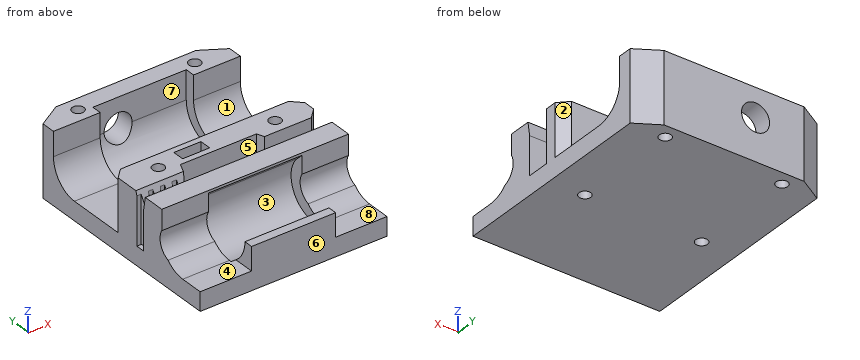
from build123d import *

# Parameters (mm, degrees)
SKETCH1_W                = 40
SKETCH1_H                = 48
BOSS_EXTRUDE1_DEPTH      = 4
BOSS_EXTRUDE2_DEPTH      = 11.15
BOSS_EXTRUDE2_DEPTH_BACK = 4
SKETCH5_W                = 40
SKETCH5_H                = 5.225
SKETCH5_W_2              = 18
SKETCH5_H_2              = 5
SKETCH5_H_3              = 6
FILLET1_DEPTH            = 40
SKETCH6_R                = 1.25
CUT_EXTRUDE4_DEPTH       = 58.214705278
CHAMFER2_SIZE            = 2
CHAMFER3_SIZE            = 3
CHAMFER3_SIZE2           = 1
CHAMFER4_SIZE            = 3
CHAMFER4_SIZE2           = 0.5
CUT_EXTRUDE6_DEPTH       = 10
CUT_EXTRUDE6_DEPTH_BACK  = 10
CUT_EXTRUDE8_REACH       = 66.292
SKETCH12_R               = 3
SKETCH13_R               = 1.5
CUT_EXTRUDE10_DEPTH      = 10.275
CUT_EXTRUDE7_DEPTH       = 1.25
CUT_EXTRUDE7_DEPTH_BACK  = 1.25
CHAMFER5_SIZE            = 5
CHAMFER5_SIZE2           = 3
CHAMFER6_SIZE            = 3
CHAMFER6_SIZE2           = 5
CUT_EXTRUDE12_DEPTH      = 46.535947422
CUT_EXTRUDE12_DEPTH_BACK = 46.535947422
SKETCH15_R               = 3.5


with BuildPart() as part:
    # Sketch1 → Boss-Extrude1 (new body)
    with BuildSketch(Plane.XY):
        with Locations((20, 14)):
            Rectangle(SKETCH1_W, SKETCH1_H)
    extrude(amount=BOSS_EXTRUDE1_DEPTH)

    # Sketch5 → Boss-Extrude2 (add, two sides: drawn at the far end of the back side and taken through both)
    with BuildSketch(Plane.XY.offset(4).offset(-BOSS_EXTRUDE2_DEPTH_BACK)):
        Polygon((0.9, 8.125), (0, 8.125), (0, 15.5), (40, 15.5), (40, 9), (28, 9), (27.357142857, 10.5), (11.081237185, 10.5), (9.763380042, 7.425), (8.800403155, 7.425), (8.500403155, 8.125), (7.531690021, 8.125), (7.231690021, 7.425), (6.221941609, 7.425), (5.921941609, 8.125), (5, 8.125), (4.7, 7.425), (3.7, 7.425), (3.4, 8.125), (2.5, 8.125), (2.2, 7.425), (1.2, 7.425), align=None)
        with Locations((20, 3.6125)):
            Rectangle(SKETCH5_W, SKETCH5_H)
        with Locations((20, -7.5)):
            Rectangle(SKETCH5_W_2, SKETCH5_H_2)
        with Locations((20, 35)):
            Rectangle(SKETCH5_W, SKETCH5_H_3)
    extrude(amount=BOSS_EXTRUDE2_DEPTH + BOSS_EXTRUDE2_DEPTH_BACK)

    # Fillet1: read off the stored shape, not the designer's step
    # Fillet1 outline → Fillet1 (add)
    with BuildSketch(Plane.YZ):
        with BuildLine():
            Line((32, 4), (32, 10))
            ThreePointArc((32, 10), (30.242640687, 5.757359313), (26, 4))
            Line((26, 4), (32, 4))
        make_face()
        with BuildLine():
            Line((1, 4), (1, 10))
            ThreePointArc((1, 10), (-0.757359313, 5.757359313), (-5, 4))
            Line((-5, 4), (1, 4))
        make_face()
    extrude(amount=FILLET1_DEPTH)

    # Sketch6 → Cut-Extrude4 (cut, through all)
    with BuildSketch(Plane.XY.offset(15.15)):
        with Locations((7.5, 35)):
            Circle(SKETCH6_R)
        with Locations((7.5, 12)):
            Circle(SKETCH6_R)
        with Locations((32.5, 35)):
            Circle(SKETCH6_R)
        with Locations((32.5, 12)):
            Circle(SKETCH6_R)
    extrude(amount=-CUT_EXTRUDE4_DEPTH, mode=Mode.SUBTRACT)

    # Chamfer2
    chamfer2_edges = [part.edges().sort_by_distance(p)[0] for p in [
        (40, 9, 9.575),
        (0, 15.5, 9.575),
        (40, 15.5, 9.575),
    ]]
    chamfer(chamfer2_edges, length=CHAMFER2_SIZE)

    # Chamfer3
    chamfer3_edges = [part.edges().sort_by_distance(p)[0] for p in [
        (4.2, 7.425, 15.15),
    ]]
    chamfer3_side = [part.faces().sort_by_distance(p)[0] for p in [
        (4.2, 7.425, 9.575),
    ]]
    chamfer(chamfer3_edges, length=CHAMFER3_SIZE, length2=CHAMFER3_SIZE2, reference=chamfer3_side[0])

    # Chamfer4
    chamfer4_edges = [part.edges().sort_by_distance(p)[0] for p in [
        (20, 6.225, 15.15),
    ]]
    chamfer4_side = [part.faces().sort_by_distance(p)[0] for p in [
        (20, 6.225, 9.575),
    ]]
    chamfer(chamfer4_edges, length=CHAMFER4_SIZE, length2=CHAMFER4_SIZE2, reference=chamfer4_side[0])

    # Sketch8 → Cut-Extrude6 (cut, two sides: drawn at the far end of the back side and taken through both)
    with BuildSketch(Plane(origin=(20, 0, 0), x_dir=(0, 0, -1), z_dir=(1, 0, 0)).offset(-CUT_EXTRUDE6_DEPTH_BACK)):
        with BuildLine():
            Line((-9, 34.1), (-18.820916768, 34.1))
            Line((-18.820916768, 34.1), (-18.820916768, 21.9))
            Line((-18.820916768, 21.9), (-9, 21.9))
            ThreePointArc((-9, 21.9), (-2.9, 28), (-9, 34.1))
        make_face()
        with BuildLine():
            Line((-18.820916768, -10.472551988), (-18.820916768, -3.194214037))
            Line((-18.820916768, -3.194214037), (-13.313351365, 2.313351365))
            ThreePointArc((-13.313351365, 2.313351365), (-3.364334852, 0.334368937), (-9, -8.1))
            Line((-9, -8.1), (-9, -10.472551988))
            Line((-9, -10.472551988), (-18.820916768, -10.472551988))
        make_face()
    extrude(amount=CUT_EXTRUDE6_DEPTH + CUT_EXTRUDE6_DEPTH_BACK, mode=Mode.SUBTRACT)

    # Cut-Extrude8: up to this face of the body (flat: up to its plane)
    cut_extrude8_end = Plane(part.part.faces().sort_by_distance((20, 15.5, 9.575))[0])
    # Sketch12 → Cut-Extrude8 (cut, up to the picked face)
    with BuildSketch(Plane(origin=(0, 38, 0), x_dir=(1, 0, 0), z_dir=(0, 1, 0)), mode=Mode.PRIVATE) as cut_extrude8_sk1:
        with Locations(Location((15.4, -9, 0), (0, 0, 270))):
            Circle(SKETCH12_R)
    cut_extrude8_tool1 = split(extrude(cut_extrude8_sk1.sketch, amount=-CUT_EXTRUDE8_REACH, mode=Mode.PRIVATE), bisect_by=cut_extrude8_end, keep=Keep.BOTH, mode=Mode.PRIVATE)
    add(cut_extrude8_tool1.solids().sort_by(Axis((15.4, 38, 9), (0, -1, 0)))[0], mode=Mode.SUBTRACT)

    # Sketch13 → Cut-Extrude10 (cut)
    with BuildSketch(Plane(origin=(0, 15.5, 0), x_dir=(1, 0, 0), z_dir=(0, 1, 0))):
        with Locations(Location((15.4, -9, 0), (0, 0, 180))):
            Circle(SKETCH13_R)
    extrude(amount=-CUT_EXTRUDE10_DEPTH, mode=Mode.SUBTRACT)

    # Sketch9 → Cut-Extrude7 (cut, two sides: drawn at the far end of the back side and taken through both)
    with BuildSketch(Plane.XZ.offset(-13).offset(-CUT_EXTRUDE7_DEPTH_BACK)):
        Polygon((12.5, 16.815347994), (18.3, 16.815347994), (18.3, 7.325684219), (15.4, 5.651368439), (12.5, 7.325684219), align=None)
    extrude(amount=CUT_EXTRUDE7_DEPTH + CUT_EXTRUDE7_DEPTH_BACK, mode=Mode.SUBTRACT)

    # Chamfer5
    chamfer5_edges = [part.edges().sort_by_distance(p)[0] for p in [
        (0, 38, 7.575),
    ]]
    chamfer5_side = [part.faces().sort_by_distance(p)[0] for p in [
        (20.225127502, 38, 7.505259415),
    ]]
    chamfer(chamfer5_edges, length=CHAMFER5_SIZE, length2=CHAMFER5_SIZE2, reference=chamfer5_side[0])

    # Chamfer6
    chamfer6_edges = [part.edges().sort_by_distance(p)[0] for p in [
        (40, 38, 7.575),
    ]]
    chamfer6_side = [part.faces().sort_by_distance(p)[0] for p in [
        (40, 5.721658913, 8.075),
    ]]
    chamfer(chamfer6_edges, length=CHAMFER6_SIZE, length2=CHAMFER6_SIZE2, reference=chamfer6_side[0])

    # Sketch15 → Cut-Extrude12 (cut, two sides: drawn at the far end of the back side and taken through both)
    with BuildSketch(Plane(origin=(20, 0, 0), x_dir=(0, 0, -1), z_dir=(1, 0, 0)).offset(-CUT_EXTRUDE12_DEPTH_BACK)):
        with Locations((-9, -2)):
            Circle(SKETCH15_R)
    extrude(amount=CUT_EXTRUDE12_DEPTH + CUT_EXTRUDE12_DEPTH_BACK, mode=Mode.SUBTRACT)


solid = part.part
CAD build for the part. Positions are in the model's coordinates, mm. Face numbers are marked on the shaded views. A direction names the side the tool comes from. Round coordinates to 2 decimals unless told otherwise and drop trailing zeros. Loops run counter-clockwise (first coordinate to the right, second up) from the corner with the lowest first, then second, coordinate; pieces in that order, holes last.
(1) Cut at D-D (y = -2). Give the cut face in (x, z), plus the area to 3 significant figures.
(2) Cut at C-C (x = 37). Give the cut face in (y, z) (3 decimals).
(3) Cut at A-A (x = 32.5). Give the cut face in (y, z) (3 decimals), plus the area to 3 significant figures.
(4) Which spindle directions (+Z, -Z, +X, -X, +Y, -Y) get a long thin tool onto all of the face, cutting with end or side? Do the marked faces 1, 2, 3, 4 and 5. Say none if no direction does.
(5) Drop flat-ended pins along their axis: pin 1 (1.3 mm diameter, centred on x = 11.5, z = 13.5, fed in from -Y); pin 2 (6 mm diameter, centred on x = 5, y = 20, fed in from +Z); pin 3 (7.5 mm diameter, centred on y = 30.5, z = 10.5, fed in from -X); pin 4 (4 mm diameter, centred on x = 34, z = 11.5, fed in from -Y). Give the stop position or say it passes through.
(6) Two-plate mould, pull along Y, no slides. Class the marked faces 6, 7 and 8: +Y half, -Y half, draft (parallel to the pull), parting line (faces both ways), or undercut.
(7) Wall check: line 1 along X through (y, z) = (12.5, 7.75); line 2 along Y through (x, z) = (35, 5) (3 decimals); line 3 along Y through (x, z) = (32.5, 11.5) (3 decimals). Give the ranges that are in metal, low to high.
(8) Cut at B-B (z = 2). Give the cut face in (x, y).
Findings below:
1. outline: (0, 0) - (40, 0) - (40, 4.8) - (30, 4.8) - (30, 2.9) - (10, 2.9) - (10, 4.8) - (0, 4.8) - close
1. area: 154 mm2
2. outline: (-10, 0) - (36.8, 0) - (36.8, 15.15) - (32, 15.15) - (32, 10) arc R6 cw to (26, 4) - (15.5, 4) - (15.5, 15.15) - (9, 15.15) - (9, 4) - (6.225, 4) - (6.225, 12.15) - (5.725, 15.15) - (1, 15.15) - (1, 10.803) arc R3.5 cw to (-0.805, 5.71) arc R6 cw to (-5, 4) - (-10, 4) - close
3. outline: (-10, 0) - (10.75, 0) - (10.75, 15.15) - (9, 15.15) - (9, 4) - (6.225, 4) - (6.225, 12.15) - (5.725, 15.15) - (1, 15.15) - (1, 10.803) arc R3.5 cw to (-0.805, 5.71) arc R6 cw to (-5, 4) - (-10, 4) - close; (13.25, 0) - (33.75, 0) - (33.75, 15.15) - (32, 15.15) - (32, 10) arc R6 cw to (26, 4) - (15.5, 4) - (15.5, 15.15) - (13.25, 15.15) - close; (36.25, 0) - (38, 0) - (38, 15.15) - (36.25, 15.15) - close
3. area: 326 mm2
4. face 1: +Z, +X, -X
4. face 2: +Z, +X
4. face 3: none
4. face 4: +Z, -X, -Y
4. face 5: +Z
5. pin 1: stops at y = 1.48
5. pin 2: stops at z = 4
5. pin 3: stops at x = 0
5. pin 4: stops at y = 1
6. face 6: -Y half
6. face 7: undercut
6. face 8: draft
7. line 1: x = 0 to 6.35, 8.65 to 12.5, 18.3 to 31.35, 33.65 to 40
7. line 2: y = -1.683 to 6.225, 9 to 15.5, 29.317 to 38
7. line 3: y = 1 to 6.225, 9 to 10.75, 13.25 to 15.5, 32 to 33.75, 36.25 to 38
8. outline: (0, -10) - (40, -10) - (40, 35) - (35, 38) - (5, 38) - (0, 35) - close; hole circle Ø2.5 at (7.5, 12); hole circle Ø2.5 at (7.5, 35); hole circle Ø2.5 at (32.5, 12); hole circle Ø2.5 at (32.5, 35)
